Part model, mm, in its own coordinate system. A direction names the side the tool comes from. Coordinates: 2 decimals unless noted, no trailing zeros. Loops run counter-clockwise (first coordinate to the right, second up) from the corner with the lowest first, then second, coordinate; pieces in that order, holes last. Notation, with made-up numbers: (18.25, 54) -> (71.25, 54) arc R6 ccw to (71.25, 64) -> close; hole circle Ø2 at (52.5, 30). An arc over 180 degrees is marked (long way). One line per question, with ' | ' between items. Start each with the question number.
1) Probe L1, parallel to Z at x = 3.25, y = 7; L2, parallel to X at y = 4, z = 10.5; L3, parallel to Z at x = 6.75, y = 6.5. List the from-to ranges inside material, lowest first. Write a range as from..to.
2) Drop flat-ended pins along their axis: pin 1 (1.7 mm diameter, centred on y = 11, z = 29.5, fed in from +X); pin 2 (5 mm diameter, centred on y = 6.97, z = 5, fed in from -X); pin 3 (0.6 mm diameter, centred on x = 3.5, z = 29.5, fed in from -Y); pin 4 (3 mm diameter, centred on x = 6.5, z = 26.5, fed in from -Y). Give the stop position or say it passes through.
3) Cut at C-C (z = 5). List the corners of the cut face in (x, y).
4) Cut at A-A (y = 4). List the corners of the cut face in (x, z), plus the area to 3 significant figures.
5) Two-plate mould, pull along Z, no slides. Class faces 1 (the face through (3, 6, 0)), 2 (the face through (3, 10, 22)), 3 (the face through (4.004, 6.047, 38.226)): released by +Z, released by -Z, zero draft, split by the parting line, or undercut.
6) 3-axis set-ups, long thin cutter, end or side, ignore diameter. For faces 4 (the face through (2, 11.97, 22)), 5 (the face through (3, 3, 22)), 6 (the face through (6, 8.667, 43)), 7 (the face through (7, 2.879, 22)), 8 (the face through (1, 0, 22)): which of +Z, -Z, +X, -X, +Y, -Y reach the whole face in a straight line?
7) Cut at D-D (x = 6.75). List the corners of the cut face in (y, z), plus the area to 3 significant figures.
8) Cut at B-B (x = 3.75). List the corners of the cut face in (y, z).
from build123d import *

# Parameters (mm, degrees)
F1_DEPTH = 45
F2_R     = 2
F3_DEPTH = 8.122212


with BuildPart() as f1:
    # F0 (on Top) → F1 (new body)
    with BuildSketch(Plane.XY):
        Polygon((0, 11.969698), (0, 0), (3, 0), (3, 5.666667), (5.121212, 5.666667), (5.121212, 2.878788), (8.121212, 2.878788), (8.121212, 8.666667), (3, 8.666667), (3, 11.969698), align=None)
    extrude(amount=F1_DEPTH)

    # F2 (on face) → F3 (cut, through all)
    with BuildSketch(Plane(origin=(0, 0, 0), x_dir=(0, -1, 0), z_dir=(-1, 0, 0))):
        with Locations((-6.969698, 5)):
            Circle(F2_R)
        with Locations((-6.969698, 40)):
            Circle(F2_R)
    extrude(amount=-F3_DEPTH, mode=Mode.SUBTRACT)


solid = f1.part
Reported:
1) L1: z = 0..3, 7..38, 42..45 | L2: x = 0..3, 5.12..8.12 | L3: z = 0..3.06, 6.94..38.06, 41.94..45
2) pin 1: stops at x = 3 | pin 2: stops at x = 0 | pin 3: stops at y = 5.67 | pin 4: stops at y = 2.88
3) outline: (0, 0) -> (3, 0) -> (3, 4.97) -> (0, 4.97) -> close; (0, 8.97) -> (3, 8.97) -> (3, 11.97) -> (0, 11.97) -> close; (5.12, 2.88) -> (8.12, 2.88) -> (8.12, 4.97) -> (5.12, 4.97) -> close
4) outline: (0, 0) -> (3, 0) -> (3, 45) -> (0, 45) -> close; (5.12, 0) -> (8.12, 0) -> (8.12, 45) -> (5.12, 45) -> close | area: 270 mm²
5) face 1: released by -Z | face 2: zero draft | face 3: undercut
6) face 4: +Z, -Z, +X, -X, +Y | face 5: +Z, -Z, -Y | face 6: +Z, -Z, +X, +Y | face 7: +Z, -Z, +X, -Y | face 8: +Z, -Z, +X, -X, -Y
7) outline: (2.88, 0) -> (8.67, 0) -> (8.67, 3.94) arc R2 cw (long way) to (8.67, 6.06) -> (8.67, 38.94) arc R2 cw (long way) to (8.67, 41.06) -> (8.67, 45) -> (2.88, 45) -> close | area: 236 mm²
8) outline: (5.67, 0) -> (8.67, 0) -> (8.67, 3.94) arc R2 cw to (5.67, 3.48) -> close; (5.67, 6.52) arc R2 cw to (8.67, 6.06) -> (8.67, 38.94) arc R2 cw to (5.67, 38.48) -> close; (5.67, 41.52) arc R2 cw to (8.67, 41.06) -> (8.67, 45) -> (5.67, 45) -> close
